from build123d import *

# Parameters (mm, degrees)
SKETCH1_W               = 140
SKETCH1_H               = 70
BASE_EXTRUDE_DEPTH      = 8
SKETCH2_W               = 70.158062676
SKETCH2_H               = 90
VERTICAL_FLANGE_DEPTH   = 8
ADUJUSTMENT_SLOT_DEPTH  = 171.106112092
HOLE_PATTERN_DEPTH      = 114.402334064
HOLE_PATTERN_DEPTH_BACK = 114.402334064
SKETCH6_R               = 5
FILLET1_R               = 3
FILLET2_R               = 3
FILLET3_R               = 3


with BuildPart() as part:
    # Sketch1 → Base Extrude (new body)
    with BuildSketch(Plane(origin=(0, 0, 0), x_dir=(1, 0, 0), z_dir=(0, 1, 0))):
        Rectangle(SKETCH1_W, SKETCH1_H)
    extrude(amount=BASE_EXTRUDE_DEPTH)

    # Sketch2 → vertical flange (add)
    with BuildSketch(Plane(origin=(70, 0, 0), x_dir=(0, 0, -1), z_dir=(1, 0, 0))):
        with Locations((0.079031338, 45)):
            Rectangle(SKETCH2_W, SKETCH2_H)
    extrude(amount=-VERTICAL_FLANGE_DEPTH)

    # Sketch3 → adujustment slot (cut, through all)
    with BuildSketch(Plane(origin=(70, 0, 0), x_dir=(0, 0, -1), z_dir=(1, 0, 0))):
        with BuildLine():
            Line((6, 60), (6, 30))
            ThreePointArc((6, 30), (0, 24), (-6, 30))
            Line((-6, 30), (-6, 60))
            ThreePointArc((-6, 60), (0, 66), (6, 60))
        make_face()
    extrude(amount=-ADUJUSTMENT_SLOT_DEPTH, mode=Mode.SUBTRACT)

    # Sketch6 → Hole_Pattern (cut, two sides: drawn at the far end of the back side and taken through both)
    with BuildSketch(Plane(origin=(0, 8, 0), x_dir=(1, 0, 0), z_dir=(0, 1, 0)).offset(-HOLE_PATTERN_DEPTH_BACK)):
        with Locations(Location((-49.427742691, 0, 0), (0, 0, 270))):
            Circle(SKETCH6_R)
        with Locations(Location((-29.427742691, 0, 0), (0, 0, 270))):
            Circle(SKETCH6_R)
        with Locations(Location((-9.427742691, 0, 0), (0, 0, 270))):
            Circle(SKETCH6_R)
        with Locations(Location((10.572257309, 0, 0), (0, 0, 270))):
            Circle(SKETCH6_R)
    extrude(amount=HOLE_PATTERN_DEPTH + HOLE_PATTERN_DEPTH_BACK, mode=Mode.SUBTRACT)

    # Fillet1
    fillet1_edges = [part.edges().sort_by_distance(p)[0] for p in [
        (-4, 0, -35),
        (0, 0, 35),
        (-70, 0, 0),
        (70, 0, -0.079031338),
    ]]
    fillet(fillet1_edges, radius=FILLET1_R)

    # Fillet2
    # the kernel refuses this fillet: 3 mm, written as the material it takes off along each edge
    with BuildSketch(Plane(origin=(-67, 3, 32), x_dir=(-1, 0, 0), z_dir=(0, 0, 1))) as fillet2_piece_1_section:
        Polygon((0, 0), (FILLET2_R, 0), (FILLET2_R, FILLET2_R), (0, FILLET2_R), align=None)
    fillet2_piece_1 = extrude(amount=FILLET2_R, mode=Mode.PRIVATE)
    fillet2_piece_1 = fillet2_piece_1 - Plane(origin=(-67, 3, 32), x_dir=(0.7071067811865475, 0.7071067811865475, 0), z_dir=(0, 0, 1)) * Sphere(FILLET2_R, mode=Mode.PRIVATE)
    add(fillet2_piece_1, mode=Mode.SUBTRACT)
    with BuildSketch(Plane(origin=(67, 3, 32), x_dir=(1, 0, 0), z_dir=(0, 0, 1))) as fillet2_piece_2_section:
        Polygon((0, 0), (FILLET2_R, 0), (FILLET2_R, -FILLET2_R), (0, -FILLET2_R), align=None)
    fillet2_piece_2 = extrude(amount=FILLET2_R, mode=Mode.PRIVATE)
    fillet2_piece_2 = fillet2_piece_2 - Plane(origin=(67, 3, 32), x_dir=(-0.7071067811865475, 0.7071067811865475, 0), z_dir=(0, 0, 1)) * Sphere(FILLET2_R, mode=Mode.PRIVATE)
    add(fillet2_piece_2, mode=Mode.SUBTRACT)
    with BuildSketch(Plane(origin=(67, 87, -32.158062676), x_dir=(0, 0, -1), z_dir=(0, 1, 0))) as fillet2_piece_3_section:
        Polygon((0, 0), (FILLET2_R, 0), (FILLET2_R, -FILLET2_R), (0, -FILLET2_R), align=None)
    fillet2_piece_3 = extrude(amount=FILLET2_R, mode=Mode.PRIVATE)
    fillet2_piece_3 = fillet2_piece_3 - Plane(origin=(67, 87, -32.158062676), x_dir=(-0.7071067811865475, 0, 0.7071067811865475), z_dir=(0, 1, 0)) * Sphere(FILLET2_R, mode=Mode.PRIVATE)
    add(fillet2_piece_3, mode=Mode.SUBTRACT)
    with BuildSketch(Plane(origin=(67, 87, 32), x_dir=(0, 1, 0), z_dir=(0, 0, 1))) as fillet2_piece_4_section:
        Polygon((0, 0), (FILLET2_R, 0), (FILLET2_R, -FILLET2_R), (0, -FILLET2_R), align=None)
    fillet2_piece_4 = extrude(amount=FILLET2_R, mode=Mode.PRIVATE)
    fillet2_piece_4 = fillet2_piece_4 - Plane(origin=(67, 87, 32), x_dir=(-0.7071067811865475, -0.7071067811865475, 0), z_dir=(0, 0, 1)) * Sphere(FILLET2_R, mode=Mode.PRIVATE)
    add(fillet2_piece_4, mode=Mode.SUBTRACT)
    with BuildSketch(Plane(origin=(67, 0, -35.158062676), x_dir=(0, 1, 0), z_dir=(-1, 0, 0)), Plane(origin=(67, 90, 35), x_dir=(0, -1, 0), z_dir=(-1, 0, 0)), Plane(origin=(67, 90, -35.158062676), x_dir=(0, 0, 1), z_dir=(-1, 0, 0))) as fillet2_piece_5:
        with BuildLine():
            CenterArc((FILLET2_R, -FILLET2_R), FILLET2_R, 90, 90)
            Line((0, -FILLET2_R), (0, 0))
            Line((0, 0), (FILLET2_R, 0))
        make_face()
    extrude(amount=12.5, mode=Mode.SUBTRACT)
    with BuildSketch(Plane(origin=(70, 90, -32.158062676), x_dir=(-1, 0, 0), z_dir=(0, 0, 1))) as fillet2_piece_6:
        with BuildLine():
            CenterArc((FILLET2_R, FILLET2_R), FILLET2_R, 180, 90)
            Line((0, FILLET2_R), (0, 0))
            Line((0, 0), (FILLET2_R, 0))
        make_face()
    extrude(amount=64.158062676, mode=Mode.SUBTRACT)
    with BuildSketch(Plane(origin=(70, 3, -35.158062676), x_dir=(-1, 0, 0), z_dir=(0, 1, 0))) as fillet2_piece_7:
        with BuildLine():
            CenterArc((FILLET2_R, FILLET2_R), FILLET2_R, 180, 90)
            Line((0, FILLET2_R), (0, 0))
            Line((0, 0), (FILLET2_R, 0))
        make_face()
    extrude(amount=84, mode=Mode.SUBTRACT)
    with BuildSketch(Plane(origin=(67, 3, -35.158062676), x_dir=(0, -1, 0), z_dir=(-1, 0, 0))) as fillet2_piece_8:
        with BuildLine():
            CenterArc((3 - FILLET2_R, FILLET2_R), FILLET2_R, 270, 90)
            Line((3, FILLET2_R), (3, 0))
            Line((3, 0), (3 - FILLET2_R, 0))
        make_face()
    revolve(axis=Axis((67, 3, -35.158062676), (0, 0, 1)), revolution_arc=90, mode=Mode.SUBTRACT)
    with BuildSketch(Plane(origin=(70, 3, 35), x_dir=(-1, 0, 0), z_dir=(0, 1, 0))) as fillet2_piece_9:
        with BuildLine():
            CenterArc((FILLET2_R, -FILLET2_R), FILLET2_R, 90, 90)
            Line((0, -FILLET2_R), (0, 0))
            Line((0, 0), (FILLET2_R, 0))
        make_face()
    extrude(amount=84, mode=Mode.SUBTRACT)
    with BuildSketch(Plane(origin=(-70, 3, 35), x_dir=(1, 0, 0), z_dir=(0, 1, 0))) as fillet2_piece_10:
        with BuildLine():
            CenterArc((FILLET2_R, FILLET2_R), FILLET2_R, 180, 90)
            Line((0, FILLET2_R), (0, 0))
            Line((0, 0), (FILLET2_R, 0))
        make_face()
    extrude(amount=12.5, mode=Mode.SUBTRACT)

    # Fillet3
    # the kernel refuses this fillet: 3 mm, written as the material it takes off along each edge
    with BuildSketch(Plane(origin=(-67, 3, -32), x_dir=(-1, 0, 0), z_dir=(0, 0, -1))) as fillet3_piece_1_section:
        Polygon((0, 0), (FILLET3_R, 0), (FILLET3_R, -FILLET3_R), (0, -FILLET3_R), align=None)
    fillet3_piece_1 = extrude(amount=FILLET3_R, mode=Mode.PRIVATE)
    fillet3_piece_1 = fillet3_piece_1 - Plane(origin=(-67, 3, -32), x_dir=(0.7071067811865475, 0.7071067811865475, 0), z_dir=(0, 0, -1)) * Sphere(FILLET3_R, mode=Mode.PRIVATE)
    add(fillet3_piece_1, mode=Mode.SUBTRACT)
    with BuildSketch(Plane(origin=(-70, 3, -35), x_dir=(1, 0, 0), z_dir=(0, 1, 0))) as fillet3_piece_2:
        with BuildLine():
            CenterArc((FILLET3_R, -FILLET3_R), FILLET3_R, 90, 90)
            Line((0, -FILLET3_R), (0, 0))
            Line((0, 0), (FILLET3_R, 0))
        make_face()
    extrude(amount=12.5, mode=Mode.SUBTRACT)


solid = part.part
Geometry check sheet. Reference: the model listing, model coordinates, mm. A direction names the side the tool comes from. Round coordinates to 2 decimals unless told otherwise and drop trailing zeros. Order: outer loops, then holes, each group sorted by start corner. A loop starts at its lowest first (then second) coordinate and runs counter-clockwise, first axis right, second up. Notation, with made-up numbers: M 48.25,27 L 59.25,27 A7 cw 59.25,40 Z; hole C 7,17.25 d7. An arc over 180 degrees is marked long. Answer in a Markdown table with one row per item.
(1) Sectioned sample at A-A, the plane z = 0. State how many separate pieces and enclosed holes the cut face has, and give its area (3 significant figures).
Responses:
| item | result |
|---|---|
| separate pieces | 6 |
| enclosed holes | 0 |
| area | 1,110 mm² |
(2) Tool access check on faces 4 (the face through (-3, 5, -35)), 5 (the face through (66, 66, 0)), 6 (the face through (-1.6, 0.86, -34.1)), 7 (the face through (20, 7, 35)), 8 (the face through (-5, 8, -8)). Record the directions out of +Z, -Z, +X, -X, +Y, -Y that give a thin tool (end or side, any length) a straight path to the whole face; none if there is none.
Responses:
| item | result |
|---|---|
| face 4 | -Z, -X, +Y, -Y |
| face 5 | +X, -X |
| face 6 | -Z, -X, -Y |
| face 7 | +Z, +X, -X, +Y, -Y |
| face 8 | +Z, -Z, -X, +Y |
(3) Draft check along Z on faces 1 (the face through (-44.47, 3.94, -0.65)), 2 (the face through (-69.14, 5.46, 34.1)), 3 (the face through (62, 56, -7)). Enter one of: released by +Z, released by -Z, zero draft, split by the parting line, or undercut.
Responses:
| item | result |
|---|---|
| face 1 | undercut |
| face 2 | released by +Z |
| face 3 | zero draft |
(4) Go/stop test with flat-tipped pins: P1, Ø1, axis at y = 43, z = -16.5, coming from the -X side; P2, Ø6, axis at x = -38, z = 4.5, coming from the +Y side; P3, Ø2.5, axis at x = 26.5, y = 6.5, coming from the -Z side. Record where each tip stops, or that it passes through.
Responses:
| item | result |
|---|---|
| P1 | stops at x = 62 |
| P2 | stops at y = 8 |
| P3 | stops at z = -35 |
(5) Scan lines: probe 1 along X at (y, z) = (3, 0); probe 2 along Y at (x, z) = (28, -11); probe 3 along Z at (x, y) = (-21, 6). Record each from-to range of solid material in increasing order. Write a range as from..to.
Responses:
| item | result |
|---|---|
| probe 1 | x = -70..-54.43, -44.43..-34.43, -24.43..-14.43, -4.43..5.57, 15.57..70 |
| probe 2 | y = 0..8 |
| probe 3 | z = -35..35 |
(6) Sectioned sample at B-B, the plane y = 48.5. Record the cut outline in (x, z).
Responses:
| item | result |
|---|---|
| outline | M 62,-35.16 L 67,-35.16 A3 ccw 70,-32.16 L 70,-6 L 62,-6 Z; M 62,6 L 70,6 L 70,32 A3 ccw 67,35 L 62,35 Z |
(7) Sectioned sample at C-C, the plane x = 9. Record the cut outline in (y, z).
Responses:
| item | result |
|---|---|
| outline | M 0,-32 A3 ccw 3,-35 L 8,-35 L 8,-4.75 L 0,-4.75 Z; M 0,4.75 L 8,4.75 L 8,35 L 3,35 A3 ccw 0,32 Z |
(8) Sectioned sample at D-D, the plane z = -7.5. Record the cut outline in (x, y).
Responses:
| item | result |
|---|---|
| outline | M -70,3 A3 ccw -67,0 L 67,0 A3 ccw 70,3 L 70,87 A3 ccw 67,90 L 62,90 L 62,8 L -70,8 Z |
